Can you work these out from the model? Positions are in its coordinate system, mm. Face numbers are marked on the shaded views. A direction names the side the tool comes from. Round coordinates to 2 decimals unless told otherwise and drop trailing zeros. Loops run counter-clockwise (first coordinate to the right, second up) from the corner with the lowest first, then second, coordinate; pieces in that order, holes last. Notation, with made-up numbers: (42.5, 81.5) -> (60.5, 81.5) arc R13 ccw to (60.5, 94.5) -> close; hole circle Ø3 at (5.25, 29). An arc over 180 degrees is marked (long way). Write each question's results on one line, items separated by ' | '.
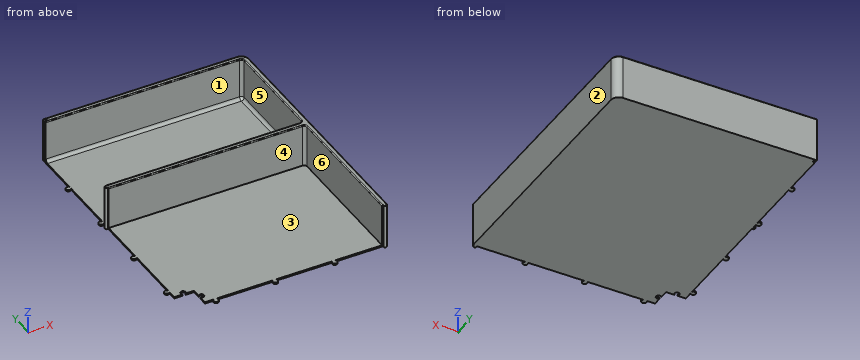
from build123d import *

# Parameters (mm, degrees)
PAD012_DEPTH           = 1.5
PAD013_DEPTH           = 43.5
FILLET005_R            = 3
FILLET006_R            = 8
SKETCH020_R            = 1.5
PAD014_DEPTH           = 45
SKETCH021_R            = 1.55
POCKET005_DEPTH        = 45.001
FILLET007_R            = 1
SKETCH022_R            = 2.5
PAD015_DEPTH           = 1.5
LINEARPATTERN005_COUNT = 3
LINEARPATTERN005_PITCH = 60
SKETCH023_R            = 2.5
PAD016_DEPTH           = 1.5
LINEARPATTERN006_COUNT = 4
LINEARPATTERN006_PITCH = 60
SKETCH024_R            = 2.5
POCKET006_DEPTH        = 45.001


with BuildPart() as part:
    # Sketch018 (on XY_Plane003 of Origin006) → Pad012 (new body)
    with BuildSketch(Plane.XY):
        Polygon((200, 240), (200, 260), (180, 260), (180, 500), (384, 500), (384, 240), align=None)
    extrude(amount=PAD012_DEPTH)

    # Sketch019 (on Face4 of Pad012) → Pad013 (join)
    with BuildSketch(Plane.XY.offset(1.5)):
        Polygon((180, 495), (180, 500), (384, 500), (384, 240), (379, 240), (379, 380), (180, 380), (180, 385), (379, 385), (379, 495), align=None)
    extrude(amount=PAD013_DEPTH)

    # Fillet005
    fillet005_edges = [part.edges().sort_by_distance(p)[0] for p in [
        (379, 380, 23.25),
        (279.5, 495, 1.5),
        (379, 495, 23.25),
        (379, 440, 1.5),
        (379, 385, 23.25),
        (279.5, 385, 1.5),
    ]]
    fillet(fillet005_edges, radius=FILLET005_R)

    # Fillet006
    fillet006_edges = [part.edges().sort_by_distance(p)[0] for p in [
        (384, 500, 23.25),
    ]]
    fillet(fillet006_edges, radius=FILLET006_R)

    # Sketch020 (on XY_Plane003 of Origin006) → Pad014 (join)
    with BuildSketch(Plane.XY):
        with Locations((381.5, 239)):
            Circle(SKETCH020_R)
        with Locations((179, 382.5)):
            Circle(SKETCH020_R)
    extrude(amount=PAD014_DEPTH)

    # Sketch021 (on XY_Plane003 of Origin006) → Pocket005 (cut, through all)
    with BuildSketch(Plane.XY):
        with Locations((181, 497.5)):
            Circle(SKETCH021_R)
    extrude(amount=POCKET005_DEPTH, mode=Mode.SUBTRACT)

    # Fillet007
    fillet007_edges = [part.edges().sort_by_distance(p)[0] for p in [
        (278, 380, 45),
        (278, 385, 45),
        (384, 366, 45),
    ]]
    fillet(fillet007_edges, radius=FILLET007_R)

    # Sketch022 (on XY_Plane003 of Origin006) → Pad015 (join)
    with BuildSketch(Plane.XY):
        with Locations((330, 238)):
            Circle(SKETCH022_R)
    pad015 = extrude(amount=PAD015_DEPTH)

    # LinearPattern005: Pad015 ×3
    with Locations(*[(-i * LINEARPATTERN005_PITCH, 0, 0) for i in range(1, LINEARPATTERN005_COUNT)]):
        add(pad015)

    # Sketch023 (on XY_Plane003 of Origin006) → Pad016 (join)
    with BuildSketch(Plane.XY):
        with Locations((178, 270)):
            Circle(SKETCH023_R)
    pad016 = extrude(amount=PAD016_DEPTH)

    # LinearPattern006: Pad016 ×4
    with Locations(*[(0, i * LINEARPATTERN006_PITCH, 0) for i in range(1, LINEARPATTERN006_COUNT)]):
        add(pad016)

    # Sketch024 (on XY_Plane003 of Origin006) → Pocket006 (cut, through all)
    with BuildSketch(Plane.XY):
        with Locations((190, 262)):
            Circle(SKETCH024_R)
        with Locations((202, 250)):
            Circle(SKETCH024_R)
    extrude(amount=POCKET006_DEPTH, mode=Mode.SUBTRACT)


solid = part.part
1. Will these pins go through, and if not, where does the flat tip stop? pin 1 (2 mm diameter, centred on y = 366, z = 33.5, fed in from -X); pin 2 (10 mm diameter, centred on x = 283, z = 32, fed in from -Y); pin 3 (0.8 mm diameter, centred on y = 256, z = 0.5, fed in from -X); pin 4 (2.5 mm diameter, centred on x = 181, y = 497.5, fed in from -Z).
Final values:
pin 1: x = 379 | pin 2: y = 380 | pin 3: x = 200 | pin 4: through
2. On a 3-axis mill with a long thin cutter (end or side, diameter ignored), from which of +Z, -Z, +X, -X, +Y, -Y can I reach the whole of each face in a straight line? I mean the marked faces 1, 2 and 3. Say none if no direction works.
Final values:
face 1: +Z, -X | face 2: +Z, -Z, +X, +Y, -Y | face 3: +Z, -X, -Y
3. If we section it at C-C (x = 353): List the corners of the cut face in (y, z) for me.
Final values:
outline: (240, 0) -> (500, 0) -> (500, 44) arc R1 ccw to (499, 45) -> (496, 45) arc R1 ccw to (495, 44) -> (495, 4.5) arc R3 cw to (492, 1.5) -> (388, 1.5) arc R3 cw to (385, 4.5) -> (385, 44) arc R1 ccw to (384, 45) -> (381, 45) arc R1 ccw to (380, 44) -> (380, 1.5) -> (240, 1.5) -> close
4. Please list where these lines run through material, in increasing order: line 1 (Y direction, x = 181, z = 34); line 2 (Y direction, x = 240.5, z = 30); line 3 (Y direction, x = 202, z = 0.5). Write a range as from..to.
Final values:
line 1: 380..385, 495..495.95, 499.05..500 | line 2: 380..385, 495..500 | line 3: 240..247.5, 252.5..500
5. We'd pull the mould along Y, two halves only. Please class the marked faces 4, 5 and 6: pulls with the +Y half, pulls with the -Y half, needs draft (parallel to the pull), parting line crosses it, or undercut.
Final values:
face 4: pulls with the -Y half | face 5: undercut | face 6: needs draft
6. If we section it at B-B (y = 294.5): List the corners of the cut face in (x, z) for me, then the cut area to 3 significant figures.
Final values:
outline: (180, 0) -> (384, 0) -> (384, 44) arc R1 ccw to (383, 45) -> (380, 45) arc R1 ccw to (379, 44) -> (379, 1.5) -> (180, 1.5) -> close | area: 523 mm2
7. If we section it at A-A (z = 8): List the corners of the cut face in (x, y) for me.
Final values:
outline: (180, 380) -> (376, 380) arc R3 cw to (379, 377) -> (379, 240) -> (380.38, 240) arc R1.5 ccw (long way) to (382.62, 240) -> (384, 240) -> (384, 492) arc R8 ccw to (376, 500) -> (180, 500) -> (180, 498.68) arc R1.55 cw (long way) to (180, 496.32) -> (180, 495) -> (376, 495) arc R3 cw to (379, 492) -> (379, 388) arc R3 cw to (376, 385) -> (180, 385) -> (180, 383.62) arc R1.5 ccw (long way) to (180, 381.38) -> close
